Build history of the part. All positions in model axes, mm. Round coordinates to 2 decimals unless told otherwise and drop trailing zeros. Write each loop counter-clockwise with the first axis right and the second up, starting at its lowest first coordinate (ties: lowest second). Pieces come first, ordered by that corner, then holes.
from build123d import *

# Parameters (mm, degrees)
SKETCH1_W           = 45
SKETCH1_H           = 204
BOSS_EXTRUDE1_DEPTH = 3
SKETCH2_W           = 10
SKETCH2_H           = 3
BOSS_EXTRUDE2_DEPTH = 3
LPATTERN1_COUNT     = 2
LPATTERN1_PITCH     = 20
SKETCH3_W           = 10
SKETCH3_H           = 3
BOSS_EXTRUDE3_DEPTH = 3
LPATTERN2_COUNT     = 2
LPATTERN2_PITCH     = 20
SKETCH4_W           = 12
SKETCH4_H           = 3
SKETCH4_W_2         = 10
BOSS_EXTRUDE4_DEPTH = 3


with BuildPart() as part:
    # Sketch1 → Boss-Extrude1 (new body)
    with BuildSketch(Plane(origin=(0, 0, 0), x_dir=(1, 0, 0), z_dir=(0, 1, 0))):
        with Locations((22.5, 102)):
            Rectangle(SKETCH1_W, SKETCH1_H)
    extrude(amount=BOSS_EXTRUDE1_DEPTH)

    # Sketch2 → Boss-Extrude2 (add)
    with BuildSketch(Plane.XY):
        with Locations((35, 1.5)):
            Rectangle(SKETCH2_W, SKETCH2_H)
    boss_extrude2 = extrude(amount=BOSS_EXTRUDE2_DEPTH)

    # LPattern1: Boss-Extrude2 ×2
    with Locations(*[(-i * LPATTERN1_PITCH, 0, 0) for i in range(1, LPATTERN1_COUNT)]):
        add(boss_extrude2)

    # Sketch3 → Boss-Extrude3 (add)
    with BuildSketch(Plane(origin=(0, 0, -204), x_dir=(-1, 0, 0), z_dir=(0, 0, -1))):
        with Locations((-35, 1.5)):
            Rectangle(SKETCH3_W, SKETCH3_H)
    boss_extrude3 = extrude(amount=BOSS_EXTRUDE3_DEPTH)

    # LPattern2: Boss-Extrude3 ×2
    with Locations(*[(-i * LPATTERN2_PITCH, 0, 0) for i in range(1, LPATTERN2_COUNT)]):
        add(boss_extrude3)

    # Sketch4 → Boss-Extrude4 (add)
    with BuildSketch(Plane(origin=(45, 0, 0), x_dir=(0, 0, -1), z_dir=(1, 0, 0))):
        with Locations((6, 1.5)):
            Rectangle(SKETCH4_W, SKETCH4_H)
        with Locations((27, 1.5)):
            Rectangle(SKETCH4_W_2, SKETCH4_H)
        with Locations((47, 1.5)):
            Rectangle(SKETCH4_W_2, SKETCH4_H)
        with Locations((67, 1.5)):
            Rectangle(SKETCH4_W_2, SKETCH4_H)
        with Locations((87, 1.5)):
            Rectangle(SKETCH4_W_2, SKETCH4_H)
        with Locations((107, 1.5)):
            Rectangle(SKETCH4_W_2, SKETCH4_H)
        with Locations((127, 1.5)):
            Rectangle(SKETCH4_W_2, SKETCH4_H)
        with Locations((147, 1.5)):
            Rectangle(SKETCH4_W_2, SKETCH4_H)
        with Locations((167, 1.5)):
            Rectangle(SKETCH4_W_2, SKETCH4_H)
        with Locations((187, 1.5)):
            Rectangle(SKETCH4_W_2, SKETCH4_H)
    extrude(amount=BOSS_EXTRUDE4_DEPTH)


solid = part.part
1) Slice it at B-B (x = 7.5). Write the cut outline in (y, z), plus the area to 3 significant figures.
Results:
outline: (0, -204) - (3, -204) - (3, 0) - (0, 0) - close
area: 612 mm2
2) Slice it at A-A (z = -75). Write the cut outline in (x, y).
Results:
outline: (0, 0) - (45, 0) - (45, 3) - (0, 3) - close
3) Wall check: L1, parallel to Z at x = 20.5, y = 0.2; L2, parallel to X at y = 2.7, z = -40. Give the ranges that are in metal, low to high.
Results:
L1: z = -204 to 0
L2: x = 0 to 45
4) Pin check, flat tips, straight feed: pin 1 Ø8 at (x, z) = (8.5, -44) entering from -Y; pin 2 Ø0.9 at (y, z) = (2, -58) entering from +X; pin 3 Ø1.5 at (x, y) = (46, 1.5) entering from -Z; pin 4 Ø1.5 at (y, z) = (2, -205) entering from -X. Stop position of each tip, or through.
Results:
pin 1: stops at y = 0
pin 2: stops at x = 45
pin 3: stops at z = -192
pin 4: stops at x = 10
